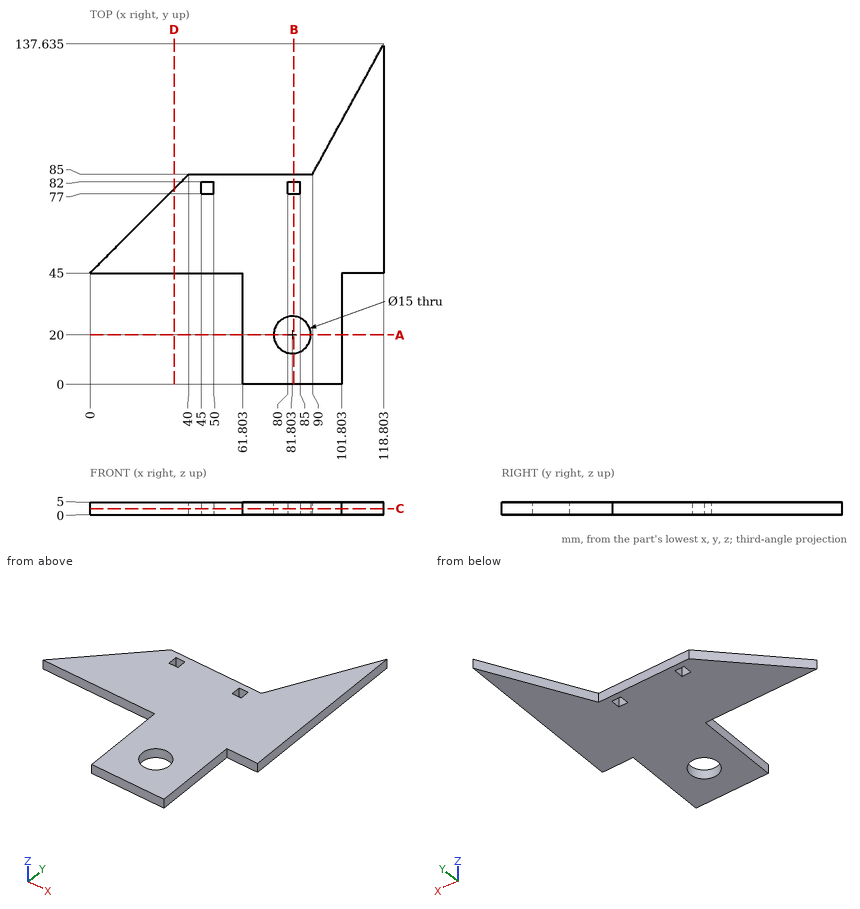
The figure shows three views and two pictorial views of one solid part (mm, origin at its lowest corner). Answer the questions. Give positions to 0.01 mm unless a question says otherwise; leave off trailing zeros. Write each loop counter-clockwise with the first axis right and the second up, starting at its lowest first coordinate (ties: lowest second). Pieces come first, ordered by that corner, then holes. Notation, with made-up numbers: M 34,67.25 L 64,67.25 A33 cw 64,103.25 Z; hole C -19,39.5 d5. An arc over 180 degrees is marked long. One line per item, written item: value. Start each with the question number.
(1) Find section B-B (x = 82.5). Determine the outline of the cut face in (y, z).
(2) Flat-ended cylindrical pins translate along their axes: pin 1 Ø2.5 at (x, z) = (47, 2.5) entering from -Y; pin 2 Ø2.5 at (y, z) = (15.5, 1.5) entering from +X; pin 3 Ø1.5 at (x, z) = (56, 4.5) entering from +Y. Find the tip coordinate at first contact, or state that the pin passes through.
(3) Find section D-D (x = 34). Determine the outline of the cut face in (y, z).
(4) Find section C-C (z = 2.45). Determine the outline of the cut face in (x, y) (1 decimal), plus the area to 3 significant figures.
(5) Find section A-A (y = 20). Determine the outline of the cut face in (x, z).
(6) Find the intervals of material crossed by line 1 (Y direction, x = 48, z = 0.4); line 2 (X direction, y = 8, z = 2.95); line 3 (X direction, y = 50, z = 3.5) (1 decimal), in increasing order.
Results below:
1. outline: M 0,0 L 12.53,0 L 12.53,5 L 0,5 Z; M 27.47,0 L 77,0 L 77,5 L 27.47,5 Z; M 82,0 L 85,0 L 85,5 L 82,5 Z
2. pin 1: stops at y = 45
2. pin 2: stops at x = 101.8
2. pin 3: stops at y = 85
3. outline: M 45,0 L 79,0 L 79,5 L 45,5 Z
4. outline: M 0,45 L 61.8,45 L 61.8,0 L 101.8,0 L 101.8,45 L 118.8,45 L 118.8,137.6 L 90,85 L 40,85 Z; hole M 45,77 L 50,77 L 50,82 L 45,82 Z; hole C 81.8,20 d15; hole M 80,77 L 85,77 L 85,82 L 80,82 Z
4. area: 6,280 mm^2
5. outline: M 61.8,0 L 74.3,0 L 74.3,5 L 61.8,5 Z; M 89.3,0 L 101.8,0 L 101.8,5 L 89.3,5 Z
6. line 1: y = 45 to 77, 82 to 85
6. line 2: x = 61.8 to 101.8
6. line 3: x = 5 to 118.8
